Source: three-view drawing plus pictorial views. Frame: mm from the lowest corner of the part. Coordinates: 2 decimals unless noted, no trailing zeros. Write each loop counter-clockwise with the first axis right and the second up, starting at its lowest first coordinate (ties: lowest second). Pieces come first, ordered by that corner, then holes.
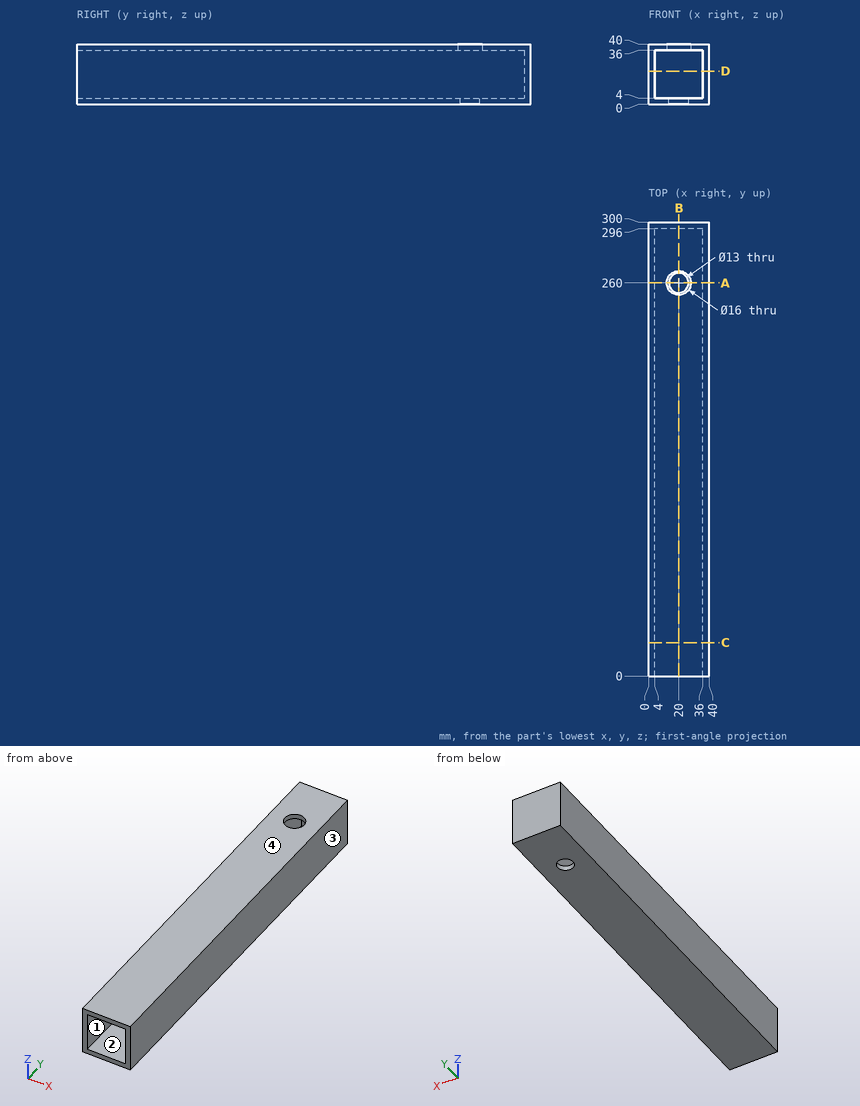
Item 1: Section query A-A, the plane y = 260. Return loops of the section in (x, z), then the cut area to 3 significant figures.
Item 2: Section query C-C, the plane y = 22. Return loops of the section in (x, z), then the cut area to 3 significant figures.
Item 3: Section query D-D, the plane z = 22. Return loops of the section in (x, y), then the cut area to 3 significant figures.
Item 4: Material intervals for line 1 (X direction, y = 260, z = 37.9); line 2 (Z direction, x = 21, y = 156), sorted ascending.
Item 5: Pull-direction query (Z, two-part tool) for the marked faces 1, 2, 3 and 4; classes: released by +Z, released by -Z, zero draft, split by the parting line, or undercut.
Item 6: Pin query (flat end, axial travel): pin 1 Ø3 at (x, z) = (33, 19.5) entering from -Y; pin 2 Ø8 at (x, y) = (20, 260) entering from +Z. Return the tip coordinate at first contact, or that it passes through.
Item 7: Section query B-B, the plane x = 20. Return loops of the section in (y, z).
The answers:
1. outline: (0, 0) - (13.5, 0) - (13.5, 4) - (4, 4) - (4, 36) - (12, 36) - (12, 40) - (0, 40) - close; (26.5, 0) - (40, 0) - (40, 40) - (28, 40) - (28, 36) - (36, 36) - (36, 4) - (26.5, 4) - close
1. area: 460 mm2
2. outline: (0, 0) - (40, 0) - (40, 40) - (0, 40) - close; hole (4, 4) - (36, 4) - (36, 36) - (4, 36) - close
2. area: 576 mm2
3. outline: (0, 0) - (4, 0) - (4, 296) - (36, 296) - (36, 0) - (40, 0) - (40, 300) - (0, 300) - close
3. area: 2,530 mm2
4. line 1: x = 0 to 12, 28 to 40
4. line 2: z = 0 to 4, 36 to 40
5. face 1: undercut
5. face 2: undercut
5. face 3: zero draft
5. face 4: released by +Z
6. pin 1: stops at y = 296
6. pin 2: passes through
7. outline: (0, 0) - (253.5, 0) - (253.5, 4) - (0, 4) - close; (0, 36) - (252, 36) - (252, 40) - (0, 40) - close; (266.5, 0) - (300, 0) - (300, 40) - (268, 40) - (268, 36) - (296, 36) - (296, 4) - (266.5, 4) - close
